Answer from the drawing. Dimensions are ordinates in mm from the lowest x, y and z of the part. A direction names the side the tool comes from. Round coordinates to 2 decimals unless told otherwise and drop trailing zeros. Loops run counter-clockwise (first coordinate to the right, second up) from the corner with the lowest first, then second, coordinate; pieces in that order, holes last. Notation, with made-up numbers: (63.25, 88.5) - (79.25, 88.5) arc R25 ccw to (79.25, 125.5) - close; hole circle Ø11 at (-31, 45.25). An arc over 180 degrees is marked (long way). Write item = value, one per line. Start each with the question number.
1) Given pin 1 Ø1.5 at (y, z) = (34, 4.5) entering from +X; pin 2 Ø4 at (x, y) = (10.5, 19.5) entering from +Z; pin 3 Ø6 at (y, z) = (10.5, 3.5) entering from +X, each flat-ended and moving along its own axis, determine where each tip first touches the part or whether it passes through.
2) Section B-B, the plane z = 10.25 is taken. Determine the outline of the cut face in (x, y), and give its area (3 significant figures).
3) Straight lines are drawn through the part: line 1 along Z through (x, y) = (8.5, 55.25); line 2 along Y through (x, z) = (8.75, 5). For each, find the intervals that lie inside material, in ascending order.
4) For a pull along Z with two mould halves and no side action, classify the marked faces 3, 4 and 5 as released by +Z, released by -Z, zero draft, split by the parting line, or undercut.
5) A tool of negligible diameter and unlimited length cuts with its end or side. For the marked faces 1 and 2, from which of +Z, -Z, +X, -X, +Y, -Y can it reach the whole face along a straight path? Write none if from no direction.
6) Section A-A, the plane y = 53 is taken. Determine the outline of the cut face in (x, z), and give its area (3 significant figures).
7) Section C-C, the plane x = 8.5 is taken. Determine the outline of the cut face in (y, z), and give its area (4 significant figures).
8) Section D-D, the plane y = 10.5 is taken. Determine the outline of the cut face in (x, z), and give its area (3 significant figures).
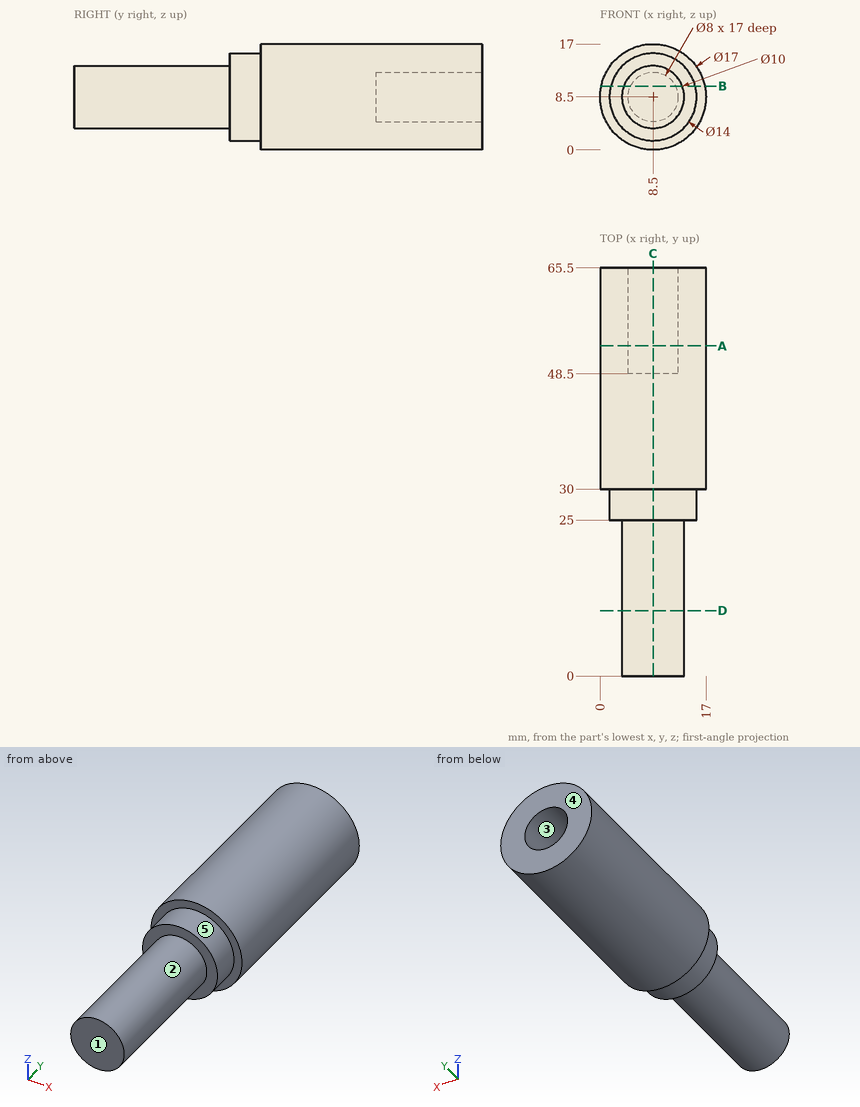
Geometry check:
q1.pin_1 = 16.35
q1.pin_2 = 13.5
q1.pin_3 = 13.08
q2.outline = (0.18, 30) - (1.72, 30) - (1.72, 25) - (3.82, 25) - (3.82, 0) - (13.18, 0) - (13.18, 25) - (15.28, 25) - (15.28, 30) - (16.82, 30) - (16.82, 65.5) - (12.1, 65.5) - (12.1, 48.5) - (4.9, 48.5) - (4.9, 65.5) - (0.18, 65.5) - close
q2.area = 770 mm2
q3.line_1 = 0 to 4.5, 12.5 to 17
q3.line_2 = 0 to 48.5
q4.face_3 = undercut
q4.face_4 = zero draft
q4.face_5 = split by the parting line
q5.face_1 = +Z, -Z, +X, -X, -Y
q5.face_2 = -Y
q6.outline = circle Ø17 at (8.5, 8.5); hole circle Ø8 at (8.5, 8.5)
q6.area = 177 mm2
q7.outline = (0, 3.5) - (25, 3.5) - (25, 1.5) - (30, 1.5) - (30, 0) - (65.5, 0) - (65.5, 4.5) - (48.5, 4.5) - (48.5, 12.5) - (65.5, 12.5) - (65.5, 17) - (30, 17) - (30, 15.5) - (25, 15.5) - (25, 13.5) - (0, 13.5) - close
q7.area = 787.5 mm2
q8.outline = circle Ø10 at (8.5, 8.5)
q8.area = 78.5 mm2
